Can you work these out from the model? Positions are in its coordinate system, mm. Round coordinates to 2 decimals unless told otherwise and drop trailing zeros. Order: outer loops, then holes, each group sorted by start corner. A loop starts at its lowest first (then second) coordinate and runs counter-clockwise, first axis right, second up.
Q1. If we section it at A-A (z = -33.5): Please give me the cut outline in (x, y), plus the area to 3 significant figures.
Q2. If we section it at C-C (z = 3): Please give me the cut outline in (x, y).
Q3. If I drill on line 1 (Z direction, x = 0, y = 1); line 2 (X direction, y = 3.25, z = -33.5); line 3 (X direction, y = 0.6, z = -33.5), over which ranges is the centre line in solid material (lowest first)?
Q4. Will these pins go through, and if not, where does the flat tip stop? P1, Ø0.6, axis at y = 2.5, z = 16, coming from the -X side; P2, Ø0.8, axis at y = 1, z = 32, coming from the +X side; P3, Ø1, axis at x = -15, y = 0.5, coming from the +Z side.
Q5. If we section it at B-B (x = 0): Please give me the cut outline in (y, z), plus the area to 3 significant figures.
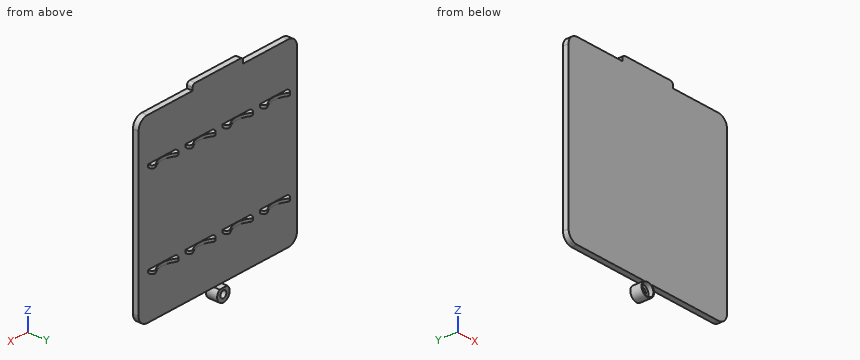
from build123d import *

# Parameters (mm, degrees)
BOSS_EXTRUDE1_DEPTH                     = 2
SKETCH2_R                               = 2.5
BOSS_EXTRUDE3_DEPTH                     = 4
SKETCH5_W                               = 11
SKETCH5_H                               = 1
EXTRUDE_THIN2_DEPTH                     = 1.5
CUT_EXTRUDE2_DEPTH                      = 49.002604096
CUT_EXTRUDE2_DEPTH_BACK                 = 49.002604096
SKETCH7_R                               = 7
FILLET2_R                               = 1
CUT_EXTRUDE3_START                      = -2
CUT_EXTRUDE3_DEPTH                      = 2
CBORE_FOR_M2_HEX_HEAD_BOLT2_D           = 2.4
CBORE_FOR_M2_HEX_HEAD_BOLT2_CBORE_D     = 4.4
CBORE_FOR_M2_HEX_HEAD_BOLT2_CBORE_DEPTH = 1.76


with BuildPart() as part:
    # Sketch1 → Boss-Extrude1 (new body)
    with BuildSketch(Plane(origin=(0, 0, 0), x_dir=(1, 0, 0), z_dir=(0, 1, 0))):
        with BuildLine():
            Line((10, -31.5), (28, -31.5))
            ThreePointArc((28, -31.5), (30.474873734, -30.474873734), (31.5, -28))
            Line((31.5, -28), (31.5, 28))
            ThreePointArc((31.5, 28), (30.474873734, 30.474873734), (28, 31.5))
            Line((28, 31.5), (-28, 31.5))
            ThreePointArc((-28, 31.5), (-30.474873734, 30.474873734), (-31.5, 28))
            Line((-31.5, 28), (-31.5, -28))
            ThreePointArc((-31.5, -28), (-30.474873734, -30.474873734), (-28, -31.5))
            Line((-28, -31.5), (-10, -31.5))
            Line((-10, -31.5), (-10, -32.5))
            ThreePointArc((-10, -32.5), (-9.707106781, -33.207106781), (-9, -33.5))
            Line((-9, -33.5), (9, -33.5))
            ThreePointArc((9, -33.5), (9.707106781, -33.207106781), (10, -32.5))
            Line((10, -32.5), (10, -31.5))
        make_face()
    extrude(amount=BOSS_EXTRUDE1_DEPTH)

    # Sketch2 → Boss-Extrude3 (add)
    with BuildSketch(Plane(origin=(0, 0, 0), x_dir=(1, 0, 0), z_dir=(0, 1, 0))):
        with Locations(Location((0, 33.5, 0), (0, 0, 233.130102354))):
            Circle(SKETCH2_R)
    extrude(amount=BOSS_EXTRUDE3_DEPTH)

    # Sketch5 → Extrude-Thin2 (add)
    with BuildSketch(Plane(origin=(0, 2, 0), x_dir=(1, 0, 0), z_dir=(0, 1, 0))):
        with Locations((-22.2, 16)):
            Rectangle(SKETCH5_W, SKETCH5_H)
        with Locations((-22.2, -16)):
            Rectangle(SKETCH5_W, SKETCH5_H)
        with Locations((-7.4, -16)):
            Rectangle(SKETCH5_W, SKETCH5_H)
        with Locations((-7.4, 16)):
            Rectangle(SKETCH5_W, SKETCH5_H)
        with Locations((7.4, -16)):
            Rectangle(SKETCH5_W, SKETCH5_H)
        with Locations((7.4, 16)):
            Rectangle(SKETCH5_W, SKETCH5_H)
        with Locations((22.2, -16)):
            Rectangle(SKETCH5_W, SKETCH5_H)
        with Locations((22.2, 16)):
            Rectangle(SKETCH5_W, SKETCH5_H)
    extrude(amount=EXTRUDE_THIN2_DEPTH)

    # Sketch7 → Cut-Extrude2 (cut, two sides: drawn at the far end of the back side and taken through both)
    with BuildSketch(Plane.XY.offset(-CUT_EXTRUDE2_DEPTH_BACK)):
        with Locations((-22.2, 9.1)):
            Circle(SKETCH7_R)
        with Locations((-7.4, 9.1)):
            Circle(SKETCH7_R)
        with Locations((7.4, 9.1)):
            Circle(SKETCH7_R)
        with Locations((22.2, 9.1)):
            Circle(SKETCH7_R)
    extrude(amount=CUT_EXTRUDE2_DEPTH + CUT_EXTRUDE2_DEPTH_BACK, mode=Mode.SUBTRACT)

    # Fillet2
    # the kernel refuses this fillet: 1 mm, written as the material it takes off along each edge
    with BuildSketch(Plane(origin=(-16.7, 3.5, 19), x_dir=(0, -1, 0), z_dir=(0, 0, -1)), Plane(origin=(-27.7, 3.5, 13), x_dir=(0, -1, 0), z_dir=(0, 0, 1)), Plane(origin=(-12.9, 3.5, 13), x_dir=(0, -1, 0), z_dir=(0, 0, 1)), Plane(origin=(-1.9, 3.5, 19), x_dir=(0, -1, 0), z_dir=(0, 0, -1)), Plane(origin=(1.9, 3.5, 13), x_dir=(0, -1, 0), z_dir=(0, 0, 1)), Plane(origin=(12.9, 3.5, 19), x_dir=(0, -1, 0), z_dir=(0, 0, -1)), Plane(origin=(16.7, 3.5, 13), x_dir=(0, -1, 0), z_dir=(0, 0, 1)), Plane(origin=(27.7, 3.5, 19), x_dir=(0, -1, 0), z_dir=(0, 0, -1)), Plane(origin=(16.7, 3.5, -19), x_dir=(0, -1, 0), z_dir=(0, 0, 1)), Plane(origin=(27.7, 3.5, -13), x_dir=(0, -1, 0), z_dir=(0, 0, -1)), Plane(origin=(12.9, 3.5, -13), x_dir=(0, -1, 0), z_dir=(0, 0, -1)), Plane(origin=(1.9, 3.5, -19), x_dir=(0, -1, 0), z_dir=(0, 0, 1)), Plane(origin=(-1.9, 3.5, -13), x_dir=(0, -1, 0), z_dir=(0, 0, -1)), Plane(origin=(-12.9, 3.5, -19), x_dir=(0, -1, 0), z_dir=(0, 0, 1)), Plane(origin=(-16.7, 3.5, -13), x_dir=(0, -1, 0), z_dir=(0, 0, -1)), Plane(origin=(-27.7, 3.5, -19), x_dir=(0, -1, 0), z_dir=(0, 0, 1))) as fillet2_piece_1:
        with BuildLine():
            CenterArc((FILLET2_R, FILLET2_R), FILLET2_R, 180, 90)
            Line((0, FILLET2_R), (0, 0))
            Line((0, 0), (FILLET2_R, 0))
        make_face()
    extrude(amount=6, mode=Mode.SUBTRACT)
    with BuildSketch(Plane(origin=(-18, 3.5, 17.302654555), x_dir=(1, 0, 0), z_dir=(0, 0, -1)), Plane(origin=(-3.2, 3.5, 17.302654555), x_dir=(1, 0, 0), z_dir=(0, 0, -1)), Plane(origin=(11.6, 3.5, 17.302654555), x_dir=(1, 0, 0), z_dir=(0, 0, -1)), Plane(origin=(26.4, 3.5, 17.302654555), x_dir=(1, 0, 0), z_dir=(0, 0, -1))) as fillet2_piece_2:
        with BuildLine():
            CenterArc((0.321061822, 1), FILLET2_R, 235.58849133, 34.41150867)
            ThreePointArc((-0.244070906, 0.175), (-0.121096827, 0.088809093), (0, 0))
            Line((0, 0), (0.321061822, 0))
        make_face()
    extrude(amount=2.605309111, mode=Mode.SUBTRACT)
    with BuildSketch(Plane(origin=(-26.4, 3.5, 17.302654555), x_dir=(0.8126870133502501, -0.5827004533479019, 0), z_dir=(0, 0, -1)), Plane(origin=(-11.6, 3.5, 17.302654555), x_dir=(0.8126870133502461, -0.5827004533479074, 0), z_dir=(0, 0, -1)), Plane(origin=(3.2, 3.5, 17.302654555), x_dir=(0.8126870133502461, -0.5827004533479074, 0), z_dir=(0, 0, -1)), Plane(origin=(18, 3.5, 17.302654555), x_dir=(0.8126870133502501, -0.5827004533479019, 0), z_dir=(0, 0, -1))) as fillet2_piece_3:
        with BuildLine():
            CenterArc((0.32177768, 0.999769883), FILLET2_R, 234.359296842, 34.41150867)
            Line((-0.260922773, 0.187082869), (0, 0))
            ThreePointArc((0, 0), (0.150162917, 0.001610821), (0.300325835, 0))
        make_face()
    extrude(amount=2.605309111, mode=Mode.SUBTRACT)
    with BuildSketch(Plane(origin=(18, 3.5, -17.302654555), x_dir=(0.8126870133502501, -0.5827004533479019, 0), z_dir=(0, 0, 1)), Plane(origin=(3.2, 3.5, -17.302654555), x_dir=(0.8126870133502461, -0.5827004533479074, 0), z_dir=(0, 0, 1)), Plane(origin=(-11.6, 3.5, -17.302654555), x_dir=(0.8126870133502461, -0.5827004533479074, 0), z_dir=(0, 0, 1)), Plane(origin=(-26.4, 3.5, -17.302654555), x_dir=(0.8126870133502501, -0.5827004533479019, 0), z_dir=(0, 0, 1))) as fillet2_piece_4:
        with BuildLine():
            CenterArc((0.32177768, -0.999769883), FILLET2_R, 91.229194488, 34.41150867)
            Line((-0.260922773, -0.187082869), (0, 0))
            ThreePointArc((0, 0), (0.150162917, -0.001610821), (0.300325835, 0))
        make_face()
    extrude(amount=2.605309111, mode=Mode.SUBTRACT)
    with BuildSketch(Plane(origin=(26.4, 3.5, -17.302654555), x_dir=(1, 0, 0), z_dir=(0, 0, 1)), Plane(origin=(11.6, 3.5, -17.302654555), x_dir=(1, 0, 0), z_dir=(0, 0, 1)), Plane(origin=(-3.2, 3.5, -17.302654555), x_dir=(1, 0, 0), z_dir=(0, 0, 1)), Plane(origin=(-18, 3.5, -17.302654555), x_dir=(1, 0, 0), z_dir=(0, 0, 1))) as fillet2_piece_5:
        with BuildLine():
            CenterArc((0.321061822, -1), FILLET2_R, 90, 34.41150867)
            ThreePointArc((-0.244070906, -0.175), (-0.121096827, -0.088809093), (0, 0))
            Line((0, 0), (0.321061822, 0))
        make_face()
    extrude(amount=2.605309111, mode=Mode.SUBTRACT)

    # Sketch8 → Cut-Extrude3 (cut)
    with BuildSketch(Plane(origin=(0, 4, 0), x_dir=(1, 0, 0), z_dir=(0, 1, 0)).offset(CUT_EXTRUDE3_START)):
        with BuildLine():
            Line((-1.5, 31.5), (1.5, 31.5))
            ThreePointArc((1.5, 31.5), (0, 31), (-1.5, 31.5))
        make_face()
    extrude(amount=CUT_EXTRUDE3_DEPTH, mode=Mode.SUBTRACT)

    # CBORE for M2 Hex Head Bolt2 (through all)
    with Locations(Plane(origin=(0, 0, 0), x_dir=(-1, 0, 0), z_dir=(0, -1, 0))):
        with Locations((0, 33.5)):
            CounterBoreHole(CBORE_FOR_M2_HEX_HEAD_BOLT2_D / 2, CBORE_FOR_M2_HEX_HEAD_BOLT2_CBORE_D / 2, CBORE_FOR_M2_HEX_HEAD_BOLT2_CBORE_DEPTH)


solid = part.part
Solution:
1. outline: (-2.5, 0) - (-2.2, 0) - (-2.2, 1.76) - (-1.2, 1.76) - (-1.2, 4) - (-2.5, 4) - close; (1.2, 1.76) - (2.2, 1.76) - (2.2, 0) - (2.5, 0) - (2.5, 4) - (1.2, 4) - close
1. area: 6.88 mm2
2. outline: (-31.5, 0) - (31.5, 0) - (31.5, 2) - (-31.5, 2) - close
3. line 1: z = -36 to -35.7, -31.3 to 33.5
3. line 2: x = -2.5 to -1.2, 1.2 to 2.5
3. line 3: x = -2.5 to -2.2, 2.2 to 2.5
4. P1: stops at x = -27.7
4. P2: stops at x = 10
4. P3: stops at z = 31.5
5. outline: (0, -36) - (4, -36) - (4, -34.7) - (1.76, -34.7) - (1.76, -35.7) - (0, -35.7) - close; (0, -31.3) - (1.76, -31.3) - (1.76, -32.3) - (4, -32.3) - (4, -31.5) - (2, -31.5) - (2, 33.5) - (0, 33.5) - close
5. area: 135 mm2
